```python
from build123d import *

# Parameters (mm, degrees)
BOSS_EXTRUDE1_DEPTH     = 160
SKETCH2_R               = 15
BOSS_EXTRUDE9_DEPTH     = 76
SKETCH6_W               = 12
SKETCH6_H               = 112.118263274
BOSS_EXTRUDE10_DEPTH    = 72
CUT_EXTRUDE6_DEPTH      = 183.439030912
CUT_EXTRUDE6_DEPTH_BACK = 183.439030912


with BuildPart() as part:
    # Sketch1 → Boss-Extrude1 (new body)
    with BuildSketch(Plane.XY):
        Polygon((0, 0), (-38, 0), (-38, -12), (-50, -12), (-50, -24), (-26, -24), (-26, -14), (26, -14), (26, -24), (50, -24), (50, -12), (38, -12), (38, 0), align=None)
    extrude(amount=BOSS_EXTRUDE1_DEPTH)

    # Sketch2 → Boss-Extrude9 (add)
    with BuildSketch(Plane(origin=(38, 0, 0), x_dir=(0, 0, -1), z_dir=(1, 0, 0))):
        with BuildLine():
            Line((-60, 0), (0, 0))
            Line((0, 0), (0, 28))
            ThreePointArc((0, 28), (-30, 58), (-60, 28))
            Line((-60, 28), (-60, 0))
        make_face()
        with Locations((-30, 28)):
            Circle(SKETCH2_R, mode=Mode.SUBTRACT)
    extrude(amount=-BOSS_EXTRUDE9_DEPTH)

    # Sketch6 → Boss-Extrude10 (add)
    with BuildSketch(Plane(origin=(0, 0, 0), x_dir=(1, 0, 0), z_dir=(0, 1, 0))):
        with Locations((0, -103.940868363)):
            Rectangle(SKETCH6_W, SKETCH6_H)
    extrude(amount=BOSS_EXTRUDE10_DEPTH)

    # Sketch7 → Cut-Extrude6 (cut, two sides: drawn at the far end of the back side and taken through both)
    with BuildSketch(Plane(origin=(0, 0, 0), x_dir=(0, 0, -1), z_dir=(1, 0, 0)).offset(-CUT_EXTRUDE6_DEPTH_BACK)):
        Polygon((-47.881736726, 52.088243848), (-160, 0), (-160, 72), (-47.881736726, 72), align=None)
    extrude(amount=CUT_EXTRUDE6_DEPTH + CUT_EXTRUDE6_DEPTH_BACK, mode=Mode.SUBTRACT)


solid = part.part
```
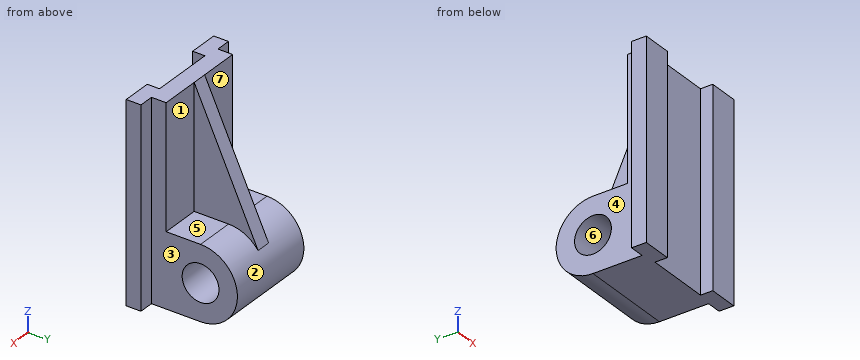
Read the model definition and answer for the solid it produces. Units are mm, in the model's axes. Face numbers are marked on the shaded views. A direction names the side the tool comes from. Coordinates: 2 decimals unless noted, no trailing zeros. Order: outer loops, then holes, each group sorted by start corner. A loop starts at its lowest first (then second) coordinate and runs counter-clockwise, first axis right, second up. Notation, with made-up numbers: (88, 61) - (124, 61) arc R32 cw to (124, 91) - close; hole circle Ø1 at (63.5, 21.25). An arc over 180 degrees is marked (long way). Answer as a JSON object with one key per item and string values. Group by question number.
Item 1: Section C-C (y = 5.5) is taken. Give the vertices of the cut face in (x, z), plus the area to 3 significant figures.
Item 2: Flat-ended cylindrical pins translate along their axes: P1, Ø6, axis at x = 44.5, z = 54.5, coming from the +Y side; P2, Ø16, axis at x = -27.5, z = 119, coming from the +Y side; P3, Ø1, axis at x = -0.5, z = 54.5, coming from the +Y side; P4, Ø12, axis at y = -8.5, z = 136.5, coming from the +X side. Find the tip coordinate at first contact, or state that the pin passes through.
Item 3: Section B-B (x = -29.5) is taken. Give the vertices of the cut face in (y, z).
Item 4: Consider probe 1 along Y at (x, z) = (1, 30); probe 2 along X at (y, z) = (-8.5, 39.5); probe 3 along X at (y, z) = (-19, 9). Determine where each line is inside the solid, lowest interval first. Write a range as from..to.
Item 5: A tool of negligible diameter and unlimited length cuts with its end or side. For the marked faces 1, 2, 3 and 4, from which of +Z, -Z, +X, -X, +Y, -Y can it reach the whole face along a straight path? Write none if from no direction.
Item 6: Section A-A (z = 30) is taken. Give the vertices of the cut face in (x, y), plus the area to 3 significant figures.
Item 7: The mould has two halves that part along Y. Classify the marked faces 5, 6 and 7: +Y half, -Y half, draft (parallel to the pull), parting line (faces both ways), or undercut.
Item 8: Section D-D (z = 90) is taken. Give the vertices of the cut face in (x, y).
Results are:
{
 "1": {"outline": "(-38, 0) - (38, 0) - (38, 60) - (6, 60) - (6, 148.16) - (-6, 148.16) - (-6, 60) - (-38, 60) - close", "area": "5,620 mm^2"},
 "2": {"P1": "stops at y = -12", "P2": "stops at y = 0", "P3": "stops at y = 49.25", "P4": "stops at x = 50"},
 "3": {"outline": "(-24, 0) - (28, 0) arc R30 ccw to (28, 60) - (0, 60) - (0, 160) - (-24, 160) - close; hole circle Ø30 at (28, 30)"},
 "4": {"probe 1": "y = -14..13, 43..58", "probe 2": "x = -38..38", "probe 3": "x = -50..-26, 26..50"},
 "5": {"face 1": "+Z, +X, +Y", "face 2": "+Y", "face 3": "+Z, -Z, +X, +Y", "face 4": "+Z, -Z, -X, +Y"},
 "6": {"outline": "(-50, -24) - (-26, -24) - (-26, -14) - (26, -14) - (26, -24) - (50, -24) - (50, -12) - (38, -12) - (38, 13) - (-38, 13) - (-38, -12) - (-50, -12) - close; (-38, 43) - (38, 43) - (38, 58) - (-38, 58) - close", "area": "3,720 mm^2"},
 "7": {"face 5": "draft", "face 6": "undercut", "face 7": "+Y half"},
 "8": {"outline": "(-50, -24) - (-26, -24) - (-26, -14) - (26, -14) - (26, -24) - (50, -24) - (50, -12) - (38, -12) - (38, 0) - (6, 0) - (6, 32.52) - (-6, 32.52) - (-6, 0) - (-38, 0) - (-38, -12) - (-50, -12) - close"}
}
